Verification items for the finished model (mm, model axes). Face numbers are marked on the shaded views. A direction names the side the tool comes from. Give positions to 0.01 mm unless a question says otherwise; leave off trailing zeros. Loops run counter-clockwise (first coordinate to the right, second up) from the corner with the lowest first, then second, coordinate; pieces in that order, holes last. Notation, with made-up numbers: (-38.75, 11.5) - (-24.75, 11.5) arc R11 cw to (-24.75, 25.5) - close; hole circle Ø1 at (0, 52). An arc over 180 degrees is marked (long way). Answer in a Markdown table with one row per item.
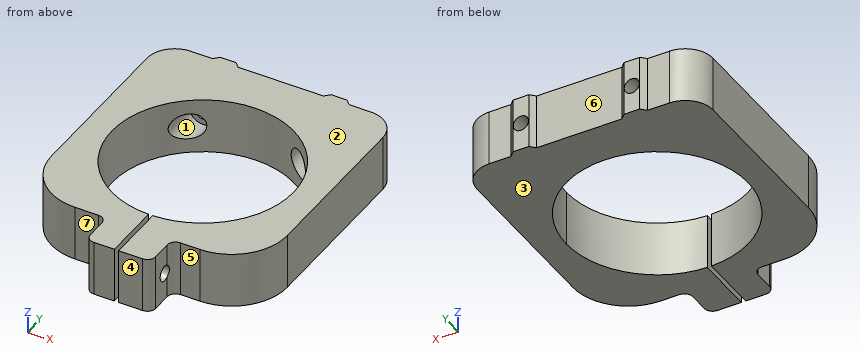
```python
from build123d import *

# Parameters (mm, degrees)
F1_DEPTH  = 10
F2_R      = 32.77
F3_DEPTH  = 10
F4_W      = 0.75
F4_H      = 80
F5_DEPTH  = 10
F6_R      = 2.7597283283
F7_DEPTH  = 25
F8_R      = 2.75
F9_DEPTH  = 17.9
F11_START = -14.2
F10_R     = 4.7926746231
F11_DEPTH = 15.7


with BuildPart() as f1:
    # F0 (on Top) → F1 (new body, symmetric)
    with BuildSketch(Plane.XY):
        with BuildLine():
            Line((-24.64, 44.1455395274), (-32.5, 44.1455395274))
            ThreePointArc((-32.5, 44.1455395274), (-39.5710678119, 41.2166073393), (-42.5, 34.1455395274))
            Line((-42.5, 34.1455395274), (-42.5, 0))
            Line((-42.5, 0), (-42.5, -25.8544604726))
            ThreePointArc((-42.5, -25.8544604726), (-36.6421356237, -39.9965960963), (-22.5, -45.8544604726))
            Line((-22.5, -45.8544604726), (-14.1281768916, -45.8544604726))
            ThreePointArc((-14.1281768916, -45.8544604726), (-12.0068565481, -46.733140129), (-11.1281768916, -48.8544604726))
            Line((-11.1281768916, -48.8544604726), (-11.1281768916, -56.0960675753))
            ThreePointArc((-11.1281768916, -56.0960675753), (-10.2494972352, -58.2173879188), (-8.1281768916, -59.0960675753))
            Line((-8.1281768916, -59.0960675753), (9.4094926704, -59.0960675753))
            ThreePointArc((9.4094926704, -59.0960675753), (11.530813014, -58.2173879188), (12.4094926704, -56.0960675753))
            Line((12.4094926704, -56.0960675753), (12.4094926704, -48.8544604726))
            ThreePointArc((12.4094926704, -48.8544604726), (13.2881723269, -46.733140129), (15.4094926704, -45.8544604726))
            Line((15.4094926704, -45.8544604726), (22.5, -45.8544604726))
            ThreePointArc((22.5, -45.8544604726), (36.6421356237, -39.9965960963), (42.5, -25.8544604726))
            Line((42.5, -25.8544604726), (42.5, 0))
            Line((42.5, 0), (42.5, 34.1455395274))
            ThreePointArc((42.5, 34.1455395274), (39.5710678119, 41.2166073393), (32.5, 44.1455395274))
            Line((32.5, 44.1455395274), (24.64, 44.1455395274))
            Line((24.64, 44.1455395274), (15.36, 44.1455395274))
            Line((15.36, 44.1455395274), (0, 44.1455395274))
            Line((0, 44.1455395274), (-15.36, 44.1455395274))
            Line((-15.36, 44.1455395274), (-20, 44.1455395274))
            Line((-20, 44.1455395274), (-24.64, 44.1455395274))
        make_face()
        Polygon((-22.84, 45.9455395274), (-24.64, 44.1455395274), (-20, 44.1455395274), (-20, 45.9455395274), align=None)
        Polygon((-20, 45.9455395274), (-20, 44.1455395274), (-15.36, 44.1455395274), (-17.16, 45.9455395274), align=None)
        Polygon((17.16, 45.9455395274), (15.36, 44.1455395274), (24.64, 44.1455395274), (22.84, 45.9455395274), (20, 45.9455395274), align=None)
    extrude(amount=F1_DEPTH, both=True)

    # F2 (on Top) → F3 (cut, symmetric)
    with BuildSketch(Plane.XY):
        with Locations((0, -4.8544604726)):
            Circle(F2_R)
    extrude(amount=F3_DEPTH, both=True, mode=Mode.SUBTRACT)

    # F4 (on Top) → F5 (cut, symmetric)
    with BuildSketch(Plane.XY):
        with Locations((0.375, -40)):
            Rectangle(F4_W, F4_H)
        with Locations((-0.375, -40)):
            Rectangle(F4_W, F4_H)
    extrude(amount=F5_DEPTH, both=True, mode=Mode.SUBTRACT)

    # F6 (on Right) → F7 (cut, symmetric)
    with BuildSketch(Plane.YZ):
        with Locations((-50.511858446, 0)):
            Circle(F6_R)
    extrude(amount=F7_DEPTH, both=True, mode=Mode.SUBTRACT)

    # F8 (on face) → F9 (cut, symmetric)
    with BuildSketch(Plane(origin=(0, 44.1455395274, 0), x_dir=(-1, 0, 0), z_dir=(0, 1, 0))):
        with Locations((20, 0)):
            Circle(F8_R)
        with Locations((-20, 0)):
            Circle(F8_R)
    extrude(amount=F9_DEPTH, both=True, mode=Mode.SUBTRACT)

    # F10 (on face) → F11 (cut)
    with BuildSketch(Plane(origin=(0, 44.1455395274, 0), x_dir=(-1, 0, 0), z_dir=(0, 1, 0)).offset(F11_START)):
        with Locations((20, 0)):
            Circle(F10_R)
        with Locations((-20, 0)):
            Circle(F10_R)
    extrude(amount=-F11_DEPTH, mode=Mode.SUBTRACT)


solid = f1.part
```
Q1. Sectioned sample at A-A (x = -9.5). Record the cut outline in (y, z).
Completed:
| item | result |
|---|---|
| outline | (-58.76, -10) - (-36.22, -10) - (-36.22, 10) - (-58.76, 10) - close; (26.51, -10) - (44.15, -10) - (44.15, 10) - (26.51, 10) - close; hole circle Ø5.52 at (-50.51, 0) |
Q2. Thickness scan on line 1 (X direction, y = -4.5, z = -3.5); line 2 (Y direction, x = 10, z = -1.75); line 3 (Y direction, x = 7, z = 0). Record the ranges inside material, lowest first.
Completed:
| item | result |
|---|---|
| line 1 | -42.5 to -32.77, 32.77 to 42.5 |
| line 2 | -59.04 to -52.65, -48.38 to -36.06, 26.35 to 44.15 |
| line 3 | -59.1 to -53.27, -47.75 to -36.87, 27.16 to 44.15 |
Q3. Sectioned sample at C-C (z = -6). Record the cut outline in (x, y).
Completed:
| item | result |
|---|---|
| outline | (-42.5, -25.85) arc R20 ccw to (-22.5, -45.85) - (-14.13, -45.85) arc R3 cw to (-11.13, -48.85) - (-11.13, -56.1) arc R3 ccw to (-8.13, -59.1) - (-0.75, -59.1) - (-0.75, -37.62) arc R32.77 cw (long way) to (0.75, -37.62) - (0.75, -59.1) - (9.41, -59.1) arc R3 ccw to (12.41, -56.1) - (12.41, -48.85) arc R3 cw to (15.41, -45.85) - (22.5, -45.85) arc R20 ccw to (42.5, -25.85) - (42.5, 34.15) arc R10 ccw to (32.5, 44.15) - (24.64, 44.15) - (22.84, 45.95) - (17.16, 45.95) - (15.36, 44.15) - (-15.36, 44.15) - (-17.16, 45.95) - (-22.84, 45.95) - (-24.64, 44.15) - (-32.5, 44.15) arc R10 ccw to (-42.5, 34.15) - close |
Q4. Draft check along Z on the marked faces 1, 2, 3 and 4. Enter one of: +Z half, -Z half, draft (parallel to the pull), parting line (faces both ways), or undercut.
Completed:
| item | result |
|---|---|
| face 1 | undercut |
| face 2 | +Z half |
| face 3 | -Z half |
| face 4 | draft |
Q5. Sectioned sample at B-B (y = 0.5). Record the cut outline in (x, z), and give its area (3 significant figures).
Completed:
| item | result |
|---|---|
| outline | (-42.5, -10) - (-32.33, -10) - (-32.33, 10) - (-42.5, 10) - close; (32.33, -10) - (42.5, -10) - (42.5, 10) - (32.33, 10) - close |
| area | 407 mm^2 |
Q6. Sectioned sample at D-D (x = -20). Record the cut outline in (y, z).
Completed:
| item | result |
|---|---|
| outline | (-45.85, -10) - (-30.81, -10) - (-30.81, 10) - (-45.85, 10) - close; (21.1, -10) - (45.95, -10) - (45.95, -2.75) - (29.95, -2.75) - (29.95, -4.79) - (21.1, -4.79) - close; (21.1, 4.79) - (29.95, 4.79) - (29.95, 2.75) - (45.95, 2.75) - (45.95, 10) - (21.1, 10) - close |
Q7. Tool access check on the marked faces 5, 6 and 7. Record the directions out of +Z, -Z, +X, -X, +Y, -Y that give a thin tool (end or side, any length) a straight path to the whole face; none if there is none.
Completed:
| item | result |
|---|---|
| face 5 | +Z, -Z, +X, -Y |
| face 6 | +Z, -Z, +Y |
| face 7 | +Z, -Z, -X, -Y |
Q8. Go/stop test with flat-tipped pins: P1, Ø6.5, axis at y = -50.51, z = 0, coming from the +X side; P2, Ø3.5, axis at y = -50.5, z = 4, coming from the -X side; P3, Ø6.5, axis at x = -28.5, z = 1.5, coming from the +Y side; P4, Ø3.5, axis at y = -50.51, z = 0, coming from the +X side. Record where each tip stops, or that it passes through.
Completed:
| item | result |
|---|---|
| P1 | x = 12.87 |
| P2 | x = -11.13 |
| P3 | y = 44.15 |
| P4 | through |
